```python
from build123d import *

# Parameters (mm, degrees)
F0_R     = 49.303083
F1_DEPTH = 89.408
F2_SIZE  = 5.08
F3_R     = 33.713024
F4_DEPTH = 70.104


with BuildPart() as f1:
    # F0 (on Top) → F1 (new body)
    with BuildSketch(Plane.XY):
        Circle(F0_R)
    extrude(amount=F1_DEPTH)

    # F2
    f2_edges = [f1.edges().sort_by_distance(p)[0] for p in [
        (-49.303083, 0, 89.408),
    ]]
    chamfer(f2_edges, length=F2_SIZE)

    # F3 (on Top) → F4 (cut)
    with BuildSketch(Plane.XY):
        Circle(F3_R)
    extrude(amount=F4_DEPTH, mode=Mode.SUBTRACT)


solid = f1.part
```
The listing builds one solid part. Answer for the finished solid, in the listing's coordinates (mm). A direction names the side the tool comes from. Coordinates: 2 decimals unless noted, no trailing zeros. Write each loop counter-clockwise with the first axis right and the second up, starting at its lowest first coordinate (ties: lowest second). Pieces come first, ordered by that corner, then holes. Notation, with made-up numbers: (-21, 37) - (6, 37) arc R29 ccw to (6, 70) - close; hole circle Ø9 at (-15.5, 58). An arc over 180 degrees is marked (long way). Return JSON: item names as keys, results as strings. Group by question number.
Q1. For a pull along Y with two mould halves and no side action, classify faces 3 (the flat face through (0, 0, 70.104)), 4 (the flat face through (-1, 1, 89.408)), 5 (the cylindrical face through (-36.34, 33.32, 41.57)) as +Y half, -Y half, draft (parallel to the pull), parting line (faces both ways), or undercut.
Q2. Find the intervals of material crossed by line 1 along Y through (x, z) = (0, 50); line 2 along Z through (x, y) = (5, 4); line 3 along X through (y, z) = (27, 62), in increasing order. Write a range as [from, to].
Q3. The part is cut by section A-A on x = 0. Write down the section's boundary in (y, z), and give its area (3 significant figures).
Q4. The part is cut by section B-B on z = 33. Write down the section's boundary in (x, y), and give its area (3 significant figures).
Q5. Which of the six approach directions +Z, -Z, +X, -X, +Y, -Y give full straight-line access (tool end or side, diameter ignored) to faces 1 (the flat face through (-12, -32, 0)), 2 (the cylindrical face through (-33.68, 1.48, 34.56))?
Q6. Flat-ended cylindrical pins translate along their axes: pin 1 Ø1.5 at (x, z) = (35.5, 26.5) entering from -Y; pin 2 Ø8 at (y, z) = (38, 73) entering from -X; pin 3 Ø1 at (y, z) = (-20, 28) entering from -X. Find the tip coordinate at first contact, or state that the pin passes through.
Evaluation:
{
 "1": {"face 3": "undercut", "face 4": "draft", "face 5": "parting line"},
 "2": {"line 1": "y = [-49.3, -33.71], [33.71, 49.3]", "line 2": "z = [70.1, 89.41]", "line 3": "x = [-41.25, -20.19], [20.19, 41.25]"},
 "3": {"outline": "(-49.3, 0) - (-33.71, 0) - (-33.71, 70.1) - (33.71, 70.1) - (33.71, 0) - (49.3, 0) - (49.3, 84.33) - (44.22, 89.41) - (-44.22, 89.41) - (-49.3, 84.33) - close", "area": "4,060 mm2"},
 "4": {"outline": "circle Ø98.61 at (0, 0); hole circle Ø67.43 at (0, 0)", "area": "4,070 mm2"},
 "5": {"face 1": "-Z, +X, -X, +Y, -Y", "face 2": "-Z"},
 "6": {"pin 1": "stops at y = -34.97", "pin 2": "stops at x = -35.7", "pin 3": "stops at x = -45.28"}
}
